from build123d import *

# Parameters (mm, degrees)
SKETCH2_R           = 18.5
SKETCH2_R_2         = 1.375
BOSS_EXTRUDE1_DEPTH = 11
SKETCH4_R           = 5
BOSS_EXTRUDE3_DEPTH = 2
SKETCH5_R           = 10
BOSS_EXTRUDE4_DEPTH = 5
FILLET1_R           = 1
CHAMFER3_SIZE       = 1
CHAMFER4_SIZE       = 1


with BuildPart() as part:
    # Sketch2 → Boss-Extrude1 (new body)
    with BuildSketch(Plane(origin=(0, 0, 0), x_dir=(1, 0, 0), z_dir=(0, 1, 0))):
        with Locations(Location((0, 0, 0), (0, 0, 270))):
            Circle(SKETCH2_R)
        with Locations(Location((0, 13.5, 0), (0, 0, 270))):
            Circle(SKETCH2_R_2, mode=Mode.SUBTRACT)
        with Locations(Location((-11.691342951, -6.75, 0), (0, 0, 270))):
            Circle(SKETCH2_R_2, mode=Mode.SUBTRACT)
        with Locations(Location((11.691342951, -6.75, 0), (0, 0, 270))):
            Circle(SKETCH2_R_2, mode=Mode.SUBTRACT)
    extrude(amount=BOSS_EXTRUDE1_DEPTH)

    # Sketch4 → Boss-Extrude3 (add)
    with BuildSketch(Plane(origin=(0, 11, 0), x_dir=(1, 0, 0), z_dir=(0, 1, 0))):
        with Locations(Location((0, 0, 0), (0, 0, 270))):
            Circle(SKETCH4_R)
    extrude(amount=BOSS_EXTRUDE3_DEPTH)

    # Sketch5 → Boss-Extrude4 (add)
    with BuildSketch(Plane(origin=(0, 13, 0), x_dir=(1, 0, 0), z_dir=(0, 1, 0))):
        with Locations(Location((0, 0, 0), (0, 0, 270))):
            Circle(SKETCH5_R)
    extrude(amount=BOSS_EXTRUDE4_DEPTH)

    # Fillet1
    fillet1_edges = [part.edges().sort_by_distance(p)[0] for p in [
        (0, 11, -5),
        (0, 13, -5),
    ]]
    fillet(fillet1_edges, radius=FILLET1_R - 0.0001)  # a hair under: the kernel refuses the full size

    # Chamfer3
    chamfer3_edges = [part.edges().sort_by_distance(p)[0] for p in [
        (11.691342951, 11, 5.375),
        (0, 11, -14.875),
        (-11.691342951, 11, 5.375),
    ]]
    chamfer(chamfer3_edges, length=CHAMFER3_SIZE)

    # Chamfer4
    chamfer4_edges = [part.edges().sort_by_distance(p)[0] for p in [
        (0, 18, -10),
        (0, 11, -18.5),
    ]]
    chamfer(chamfer4_edges, length=CHAMFER4_SIZE)


solid = part.part
Verification items for the finished model (mm, model axes). A direction names the side the tool comes from. Give positions to 0.01 mm unless a question says otherwise; leave off trailing zeros. Order: outer loops, then holes, each group sorted by start corner. A loop starts at its lowest first (then second) coordinate and runs counter-clockwise, first axis right, second up. Notation, with made-up numbers: M 26.5,-37 L 79.5,-37 A22 cw 79.5,-28 Z; hole C -7,-8.5 d9. An arc over 180 degrees is marked long. Answer as a JSON object with one key per item and string values. Group by question number.
1) Depth check by flat-ended pin: pin 1 Ø2 at (x, y) = (5.5, 5.5) entering from -Z; pin 2 Ø4 at (y, z) = (7, -12.5) entering from +X; pin 3 Ø1 at (x, z) = (12.5, 2) entering from +Y. Enter the tip coordinate at first touch or a pass-through.
2) Access from +Z, -Z, +X, -X, +Y, -Y to the whole of each face (thin tool, end or side, straight path). Record for faces 4 (the face through (0, 18, 0)), 5 (the face through (0, 11, 8)).
3) Cross-section at D-D (z = 6.75). Give the number of separate pieces and of enclosed holes in the cut face, then the cut area to 3 significant figures.
4) Mould release check, pull along Z, two halves, no side actions. Record for faces 1 (the face through (0, 0, 0)), 2 (the face through (13.055, 4.93, 6.571)), 3 (the face through (-9.76, 14.97, -2.17)): released by +Z, released by -Z, zero draft, split by the parting line, or undercut.
5) Scan lines: line 1 along Y through (x, z) = (8, -0.5); line 2 along X through (y, z) = (2.5, 6.75); line 3 along Y through (x, z) = (14, -4). Record each from-to range of solid material in increasing order. Write a range as [from, to].
6) Cross-section at C-C (y = 15.5). Enter the section's corners in (x, z), then the cut area to 3 significant figures.
Result sheet:
{
 "1": {"pin 1": "stops at z = -17.94", "pin 2": "stops at x = 15.23", "pin 3": "stops at y = 11"},
 "2": {"face 4": "+Z, -Z, +X, -X, +Y", "face 5": "none"},
 "3": {"separate pieces": "4", "enclosed holes": "0", "area": "388 mm2"},
 "4": {"face 1": "zero draft", "face 2": "undercut", "face 3": "split by the parting line"},
 "5": {"line 1": "y = [0, 11], [13, 18]", "line 2": "x = [-17.22, -13.07], [-10.32, 10.32], [13.07, 17.22]", "line 3": "y = [0, 11]"},
 "6": {"outline": "C 0,0 d20", "area": "314 mm2"}
}
